Read the model definition and answer for the solid it produces. Units are mm, in the model's axes. Coordinates: 2 decimals unless noted, no trailing zeros. Order: outer loops, then holes, each group sorted by start corner. A loop starts at its lowest first (then second) coordinate and runs counter-clockwise, first axis right, second up. Notation, with made-up numbers: (-29.75, 56.5) - (-3.75, 56.5) arc R17 cw to (-3.75, 61.5) - close; hole circle Ø1 at (-40, 67.25). An arc over 180 degrees is marked (long way). Use one line per item in the form item = value.
Autodesk Inventor part; units mm, degrees
ref_plane "YZ Plane" through (0, 0, 0) normal (1, 0, 0) x (0, 1, 0)
ref_plane "XZ Plane" through (0, 0, 0) normal (0, 1, 0) x (-1, 0, 0)
ref_plane "XY Plane" through (0, 0, 0) normal (0, 0, 1) x (1, 0, 0)
sketch "Sketch1" plane through (0, 0, 0) normal (1, 0, 0) x (0, 1, 0)
  line L0 (11.2555, 71.2167) -> (-70.0245, 71.2167)
  line L1 (-70.0245, 71.2167) -> (-70.0245, -10.0633)
  line L2 (-70.0245, -10.0633) -> (11.2555, -10.0633)
  line L3 (11.2555, -10.0633) -> (11.2555, 71.2167)
  point P0 (0, 0)
  dimension "d0" = 81.28
  dimension "d1" = 81.28
extrude "Extrusion1" add sketch "Sketch1" along normal blind 3.175
sketch "Sketch2" plane through (3.175, 0, 0) normal (1, 0, 0) x (0, 0, -1)
  circle A0 centre (-30.5767, -29.3845) radius 9.525
  line L0 (10.0633, 11.2555) -> (-71.2167, 11.2555)
  line L1 (-71.2167, 11.2555) -> (-71.2167, -70.0245)
  circle A1 centre (-10.2567, -10.9695) radius 2.3495
  circle A2 centre (-50.8967, -47.7995) radius 2.3495
  line L2 (-71.2167, -70.0245) -> (10.0633, -70.0245)
  line L3 (10.0633, -70.0245) -> (10.0633, 11.2555)
  point P0 (0, 0)
  dimension "d4" = 19.05
  dimension "d5" = 40.64
  dimension "d6" = 40.64
  dimension "d9" = 4.699
  dimension "d10" = 4.699
  dimension "d11" = 20.32
  dimension "d12" = 22.225
  dimension "d13" = 22.225
  dimension "d14" = 20.32
extrude "Extrusion2" cut sketch "Sketch2" against normal blind 3.175 contours A0 | A1 | A2
properties part number "Guard Plate"
(1) The mould has two halves that part along Y. Classify faces 1 (the flat face through (2, -30, -10.063)), 2 (the flat face through (2, 11.256, 30)), 3 (the cylindrical face through (1.61, -35.18, 38.135)): +Y half, -Y half, draft (parallel to the pull), parting line (faces both ways), or undercut.
Answer list:
face_1 = draft
face_2 = +Y half
face_3 = undercut
(2) Section C-C, the plane z = 10 is taken. Write down the section's boundary in (x, y) (1 decimal), then the cut area to 3 significant figures.
Answer list:
outline = (0, -70) - (3.2, -70) - (3.2, -13.3) - (0, -13.3) - close; (0, -8.6) - (3.2, -8.6) - (3.2, 11.3) - (0, 11.3) - close
area = 243 mm2
(3) Section A-A, the plane y = -27.5 is taken. Write down the section's boundary in (x, z) (3 decimals).
Answer list:
outline = (0, -10.063) - (3.175, -10.063) - (3.175, 21.24) - (0, 21.24) - close; (0, 39.913) - (3.175, 39.913) - (3.175, 71.217) - (0, 71.217) - close
(4) Given pin 1 Ø3 at (y, z) = (-14.5, 39) entering from -X; pin 2 Ø11.5 at (y, z) = (-29.38, 30.58) entering from +X, each flat-ended and moving along its own axis, determine where each tip first touches the part or whether it passes through.
Answer list:
pin_1 = 0
pin_2 = through
(5) Section B-B, the plane x = 0.5 is taken. State how many separate pieces and enclosed holes the cut face has, then the cut area to 3 significant figures.
Answer list:
separate_pieces = 1
enclosed_holes = 3
area = 6,290 mm2
(6) Straight lines are drawn through the part: L1, parallel to Z at x = 0.5, y = -35.5; L2, parallel to Y at x = 2.35, z = 32; L3, parallel to Z at x = 2.1, y = -10.5. For each, find the intervals that lie inside material, in ascending order.
Answer list:
L1 = -10.06 to 23.27, 37.88 to 71.22
L2 = -70.02 to -38.8, -19.97 to 11.26
L3 = -10.06 to 7.95, 12.56 to 71.22
